from build123d import *

# Parameters (mm, degrees)
F0_W     = 80
F0_H     = 48
F1_DEPTH = 25
F2_W     = 19.5
F2_H     = 10
F3_DEPTH = 25.001
F4_R     = 7.5
F5_DEPTH = 25.001
F6_R     = 5.5
F6_R_2   = 4
F7_DEPTH = 25
F8_DEPTH = 38.001


with BuildPart() as f1:
    # F0 (on Right) → F1 (new body)
    with BuildSketch(Plane.YZ):
        Rectangle(F0_W, F0_H)
    extrude(amount=-F1_DEPTH)

    # F2 (on face) → F3 (cut, through all)
    with BuildSketch(Plane.YZ):
        with Locations((-30.25, 19)):
            Rectangle(F2_W, F2_H)
        with Locations((30.25, 19)):
            Rectangle(F2_W, F2_H)
    extrude(amount=-F3_DEPTH, mode=Mode.SUBTRACT)

    # F4 (on face) → F5 (cut, through all)
    with BuildSketch(Plane.YZ):
        with Locations((0, 4)):
            Circle(F4_R)
    extrude(amount=-F5_DEPTH, mode=Mode.SUBTRACT)

    # F6 (on face) → F7 (cut)
    with BuildSketch(Plane.XY.offset(14)):
        with Locations((-12.5, 30)):
            Circle(F6_R)
        with Locations((-12.5, 30)):
            Circle(F6_R_2, mode=Mode.SUBTRACT)
        with Locations((-12.5, -30)):
            Circle(F6_R)
        with Locations((-12.5, -30)):
            Circle(F6_R_2, mode=Mode.SUBTRACT)
    extrude(amount=-F7_DEPTH, mode=Mode.SUBTRACT)

    # F8 (cut, through all): faces of the model
    f8_faces = [f1.faces().sort_by_distance(p)[0] for p in [
        (-12.5, 30, 14),
        (-12.5, -30, 14),
    ]]
    extrude(f8_faces, amount=-F8_DEPTH, mode=Mode.SUBTRACT)


solid = f1.part
Could you check a few things on this model? Use its own coordinates, in mm. A direction names the side the tool comes from. Coordinates: 2 decimals unless noted, no trailing zeros. Order: outer loops, then holes, each group sorted by start corner. A loop starts at its lowest first (then second) coordinate and runs counter-clockwise, first axis right, second up. Notation, with made-up numbers: (22, -31.75) -> (37, -31.75) arc R19 ccw to (37, -3.75) -> close; hole circle Ø5 at (-14.5, -24.75). An arc over 180 degrees is marked (long way). One line per item, written item: value. Start each with the question number.
1) If I drill on L1, parallel to Y at x = -12.5, z = -4.5; L2, parallel to Y at x = -12.5, z = 4.5; L3, parallel to Y at x = -9.75, z = -22, over which ranges is the centre line in solid material (lowest first)? Write a range as [from, to].
2) Imagine slicing it at B-B on z = -2.5. List the corners of the cut face in (x, y) for me, plus the area to 3 significant figures.
3) I'm going to push flat-ended pins straight in: pin 1 (13 mm diameter, centred on x = -12.5, y = 30, fed in from -Z); pin 2 (5.5 mm diameter, centred on x = -11.5, y = 31, fed in from +Z); pin 3 (13 mm diameter, centred on x = -12.5, y = -30, fed in from +Z); pin 4 (1 mm diameter, centred on x = -22, z = 18.5, fed in from +Y). Where does each tip first touch, or does it pass through?
4) Which directions (+Z, -Z, +X, -X, +Y, -Y) give clear straight access to the entire face, cutting with the end or side of a thin tool? Please do faces 5 (the flat face through (-12, 20.5, 19)), 6 (the flat face through (-12, -20.5, 19)), 7 (the cylindrical face through (-7.254, -28.348, 1.675)).
5) Imagine slicing it at C-C on y = 30. List the corners of the cut face in (x, z) for me.
6) We'd pull the mould along Z, two halves only. Please class faces 1 (the flat face through (-12, -1, -24)), 2 (the flat face through (-6.8, -30.4, 14)), 3 (the cylindrical face through (-12.325, -0.976, 11.436)), 4 (the flat face through (-12, 40, -5)): +Z half, -Z half, draft (parallel to the pull), parting line (faces both ways), or undercut.
7) Imagine slicing it at D-D on x = -19. List the corners of the cut face in (y, z) for me.
8) Imagine slicing it at A-A on x = -12.5. List the corners of the cut face in (y, z) for me, plus the area to 3 significant figures.
Answer list:
1. L1: y = [-40, -35.5], [-24.5, 24.5], [35.5, 40]
1. L2: y = [-40, -35.5], [-24.5, -7.48], [7.48, 24.5], [35.5, 40]
1. L3: y = [-40, -32.9], [-27.1, 27.1], [32.9, 40]
2. outline: (-25, -40) -> (0, -40) -> (0, -3.74) -> (-25, -3.74) -> close; (-25, 3.74) -> (0, 3.74) -> (0, 40) -> (-25, 40) -> close; hole circle Ø11 at (-12.5, -30); hole circle Ø11 at (-12.5, 30)
2. area: 1,620 mm2
3. pin 1: stops at z = -24
3. pin 2: stops at z = -11
3. pin 3: stops at z = 14
3. pin 4: stops at y = 20.5
4. face 5: +Z, +X, -X, +Y
4. face 6: +Z, +X, -X, -Y
4. face 7: +Z
5. outline: (-25, -24) -> (-16.5, -24) -> (-16.5, -11) -> (-18, -11) -> (-18, 14) -> (-25, 14) -> close; (-8.5, -24) -> (0, -24) -> (0, 14) -> (-7, 14) -> (-7, -11) -> (-8.5, -11) -> close
6. face 1: -Z half
6. face 2: +Z half
6. face 3: undercut
6. face 4: draft
7. outline: (-40, -24) -> (40, -24) -> (40, 14) -> (20.5, 14) -> (20.5, 24) -> (-20.5, 24) -> (-20.5, 14) -> (-40, 14) -> close; hole circle Ø15 at (0, 4)
8. outline: (-40, -24) -> (-34, -24) -> (-34, -11) -> (-35.5, -11) -> (-35.5, 14) -> (-40, 14) -> close; (-26, -24) -> (26, -24) -> (26, -11) -> (24.5, -11) -> (24.5, 14) -> (20.5, 14) -> (20.5, 24) -> (-20.5, 24) -> (-20.5, 14) -> (-24.5, 14) -> (-24.5, -11) -> (-26, -11) -> close; (34, -24) -> (40, -24) -> (40, 14) -> (35.5, 14) -> (35.5, -11) -> (34, -11) -> close; hole circle Ø15 at (0, 4)
8. area: 2,520 mm2
